Check sheet for the drawn part. Datum: minimum x, y, z corner. Units: mm. A direction names the side the tool comes from. Coordinates: 2 decimals unless noted, no trailing zeros. Order: outer loops, then holes, each group sorted by start corner. A loop starts at its lowest first (then second) coordinate and runs counter-clockwise, first axis right, second up.
Q1. Set-up check for the marked faces 1 and 2: record each of +Z, -Z, +X, -X, +Y, -Y from which the full face is reachable in a straight line by a thin tool's end or side.
Q2. Cross-section at D-D, the plane x = 37. Record the boundary of the cut face in (y, z), and give its area (3 significant figures).
Q3. Thickness scan on line 1 (X direction, y = 49.5, z = 47); line 2 (Z direction, x = 37, y = 35); line 3 (Y direction, x = 55, z = 63.5). Record the ranges inside material, lowest first.
Q4. Cross-section at C-C, the plane y = 65. Record the boundary of the cut face in (x, z), and give its area (3 significant figures).
Q5. Depth check by flat-ended pin: P1, Ø4, axis at y = 29.5, z = 65.5, coming from the +X side; P2, Ø8, axis at x = 60, y = 61, coming from the -Z side; P3, Ø5.5, axis at y = 41.5, z = 65, coming from the -X side; P4, Ø8, axis at x = 62, y = 62, coming from the -Z side. Enter the tip coordinate at first touch or a pass-through.
Q6. Cross-section at B-B, the plane z = 6.5. Record the boundary of the cut face in (x, y).
Q7. Cross-section at A-A, the plane y = 56. Record the boundary of the cut face in (x, z) (3 decimals).
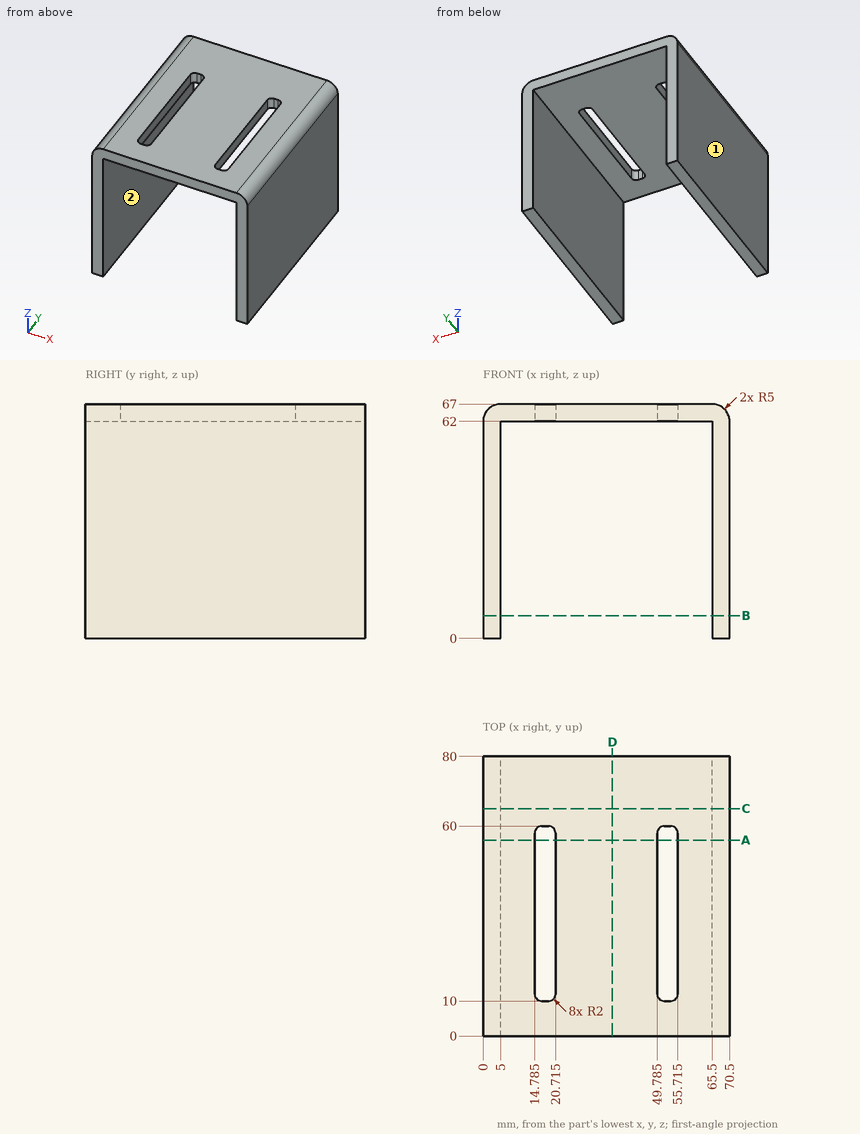
Check values:
1. face 1: +Z, -Z, -X, +Y, -Y
1. face 2: -Z, +Y, -Y
2. outline: (0, 62) - (80, 62) - (80, 67) - (0, 67) - close
2. area: 400 mm2
3. line 1: x = 0 to 5, 65.5 to 70.5
3. line 2: z = 62 to 67
3. line 3: y = 0 to 10.47, 59.53 to 80
4. outline: (0, 0) - (5, 0) - (5, 62) - (65.5, 62) - (65.5, 0) - (70.5, 0) - (70.5, 62) arc R5 ccw to (65.5, 67) - (5, 67) arc R5 ccw to (0, 62) - close
4. area: 962 mm2
5. P1: stops at x = 70.27
5. P2: stops at z = 62
5. P3: stops at x = 0.01
5. P4: stops at z = 0
6. outline: (0, 0) - (5, 0) - (5, 80) - (0, 80) - close; (65.5, 0) - (70.5, 0) - (70.5, 80) - (65.5, 80) - close
7. outline: (0, 0) - (5, 0) - (5, 62) - (14.785, 62) - (14.785, 67) - (5, 67) arc R5 ccw to (0, 62) - close; (20.715, 62) - (49.785, 62) - (49.785, 67) - (20.715, 67) - close; (55.715, 62) - (65.5, 62) - (65.5, 0) - (70.5, 0) - (70.5, 62) arc R5 ccw to (65.5, 67) - (55.715, 67) - close
